Job drawing, mm, ordinate dimensions from the low corner. One solid piece. A direction names the side the tool comes from. Give positions to 0.01 mm unless a question says otherwise; leave off trailing zeros. Order: outer loops, then holes, each group sorted by start corner. A loop starts at its lowest first (then second) coordinate and runs counter-clockwise, first axis right, second up. Notation, with made-up numbers: M 56.25,53.5 L 104.25,53.5 A4 ccw 104.25,58.5 Z; hole C -0.75,-40 d7. An arc over 180 degrees is marked long. One line per question, with ' | ' between items.
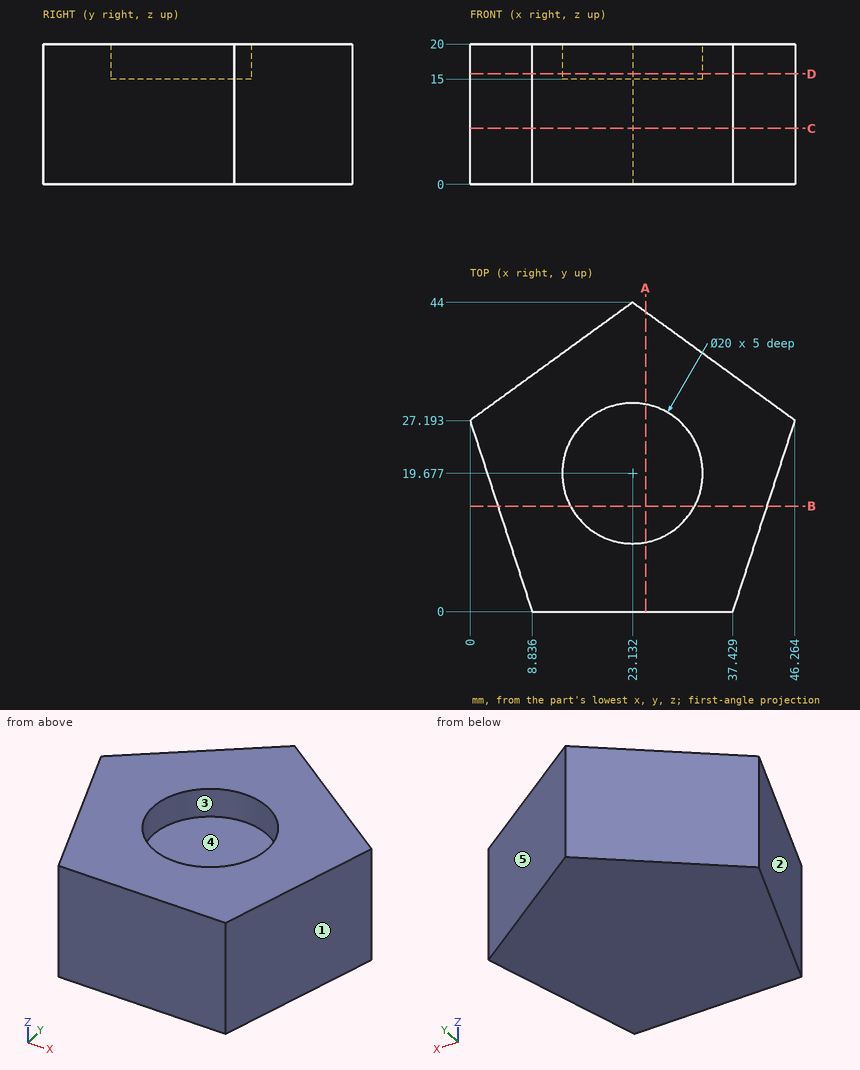
1. Drop flat-ended pins along their axis: pin 1 (3 mm diameter, centred on y = 6, z = 16, fed in from -X); pin 2 (1 mm diameter, centred on x = 10.5, z = 10.5, fed in from +Y) (1 decimal); pin 3 (5 mm diameter, centred on y = 19, z = 5, fed in from +X) (1 decimal); pin 4 (2 mm diameter, centred on x = 14, y = 39, fed in from -Z). Give the stop position or say it passes through.
Worked out:
pin 1: stops at x = 6.4 | pin 2: stops at y = 35.2 | pin 3: stops at x = 44.4 | pin 4: passes through
2. Probe L1, parallel to Z at x = 16, y = 24; L2, parallel to X at y = 31.5, z = 19 (1 decimal); L3, parallel to Y at x = 16.5, z = 3.5. List the from-to ranges inside material, lowest first. Write a range as from..to.
Worked out:
L1: z = 0..15 | L2: x = 5.9..40.3 | L3: y = 0..39.18
3. Mould opens along X. For the marked faces 1, 2 and 3 say: released by +X, released by -X, zero draft, split by the parting line, or undercut.
Worked out:
face 1: released by +X | face 2: released by -X | face 3: undercut
4. Slice it at D-D on z = 15.75. Give the cut face in (x, y) (1 decimal), then the cut area to 3 significant figures.
Worked out:
outline: M 0,27.2 L 8.8,0 L 37.4,0 L 46.3,27.2 L 23.1,44 Z; hole C 23.1,19.7 d20 | area: 1,090 mm2
5. Tool access for the marked faces 4 and 5: list every direction of +Z, -Z, +X, -X, +Y, -Y with a clear straight run to the whole face (end or side of a thin tool).
Worked out:
face 4: +Z | face 5: +Z, -Z, +X, +Y
6. Slice it at A-A on x = 25. Give the cut face in (y, z).
Worked out:
outline: M 0,0 L 42.64,0 L 42.64,20 L 29.5,20 L 29.5,15 L 9.85,15 L 9.85,20 L 0,20 Z
7. Slice it at B-B on y = 15. Give the cut face in (x, z).
Worked out:
outline: M 3.96,0 L 42.3,0 L 42.3,20 L 31.97,20 L 31.97,15 L 14.29,15 L 14.29,20 L 3.96,20 Z
8. Slice it at C-C on z = 8. Give the cut face in (x, y) (1 decimal).
Worked out:
outline: M 0,27.2 L 8.8,0 L 37.4,0 L 46.3,27.2 L 23.1,44 Z
